Model file for the job. Use its own axes, mm. Face numbers are marked on the shaded views. A direction names the side the tool comes from. Round coordinates to 2 decimals unless told otherwise and drop trailing zeros. Order: outer loops, then holes, each group sorted by start corner. A loop starts at its lowest first (then second) coordinate and runs counter-clockwise, first axis right, second up. Notation, with made-up numbers: (56, 72) - (89, 72) arc R29 cw to (89, 96) - close; hole circle Ø7 at (-27.5, -22.5). An arc over 180 degrees is marked (long way). Answer as CSV lines item,"result". Start each with the question number.
1. Band-saw the part on B-B on y = 3.75. List the corners of the cut face in (x, z), then the cut area to 3 significant figures.
2. Pin check, flat tips, straight feed: pin 1 Ø6 at (x, y) = (2, -1.5) entering from +Z; pin 2 Ø1.5 at (x, y) = (-2.5, 1) entering from +Z. Stop position of each tip, or through.
3. Band-saw the part on C-C on z = 10.25. List the corners of the cut face in (x, y), then the cut area to 3 significant figures.
4. Band-saw the part on A-A on z = 8. List the corners of the cut face in (x, y).
5. Band-saw the part on D-D on x = -3.5. List the corners of the cut face in (y, z), then the cut area to 3 significant figures.
6. Wall check: line 1 along Y through (x, z) = (0, 9.8); line 2 along Y through (x, z) = (1, 7.5); line 3 along X through (y, z) = (0, 9.7). Give the ranges that are in metal, low to high. Write a range as [from, to].
7. Pull direction Y, two halves, no side cores. Call the marked faces 1, 2 and 3: released by +Y, released by -Y, zero draft, split by the parting line, or undercut.
8. 3-axis set-ups, long thin cutter, end or side, ignore diameter. For the marked faces 4 and 5: which of +Z, -Z, +X, -X, +Y, -Y reach the whole face in a straight line?
```python
from build123d import *

# Parameters (mm, degrees)
F0_W          = 10
F0_H          = 10
F1_DEPTH      = 25
F1_DEPTH_BACK = 5
F4_W          = 10
F4_H          = 5.4510665399
F5_DEPTH      = 25
F5_DEPTH_BACK = 25


with BuildPart() as f1:
    # F0 (on Top) → F1 (new body, two sides)
    with BuildSketch(Plane.XY) as f1_sk:
        Rectangle(F0_W, F0_H)
    extrude(amount=F1_DEPTH)
    extrude(f1_sk.sketch, amount=-F1_DEPTH_BACK)

    # F2 (on Front) → F3 (revolve, cut)
    with BuildSketch(Plane.XZ):
        Polygon((2.55, 8.6417774172), (2.55, 25), (0, 25), (0, 5), align=None)
    revolve(axis=Axis((0, 0, 15), (0, 0, -1)), mode=Mode.SUBTRACT)

    # F4 (on Front) → F5 (cut, two sides)
    with BuildSketch(Plane.XZ) as f5_sk:
        with BuildLine():
            ThreePointArc((-5, 11.7330665399), (0.3429792874, 10.3044447979), (5, 7.3210665399))
            Line((5, 7.3210665399), (5, 25))
            Line((5, 25), (-5, 25))
            Line((-5, 25), (-5, 11.7330665399))
        make_face()
        with Locations((0, -2.2744667301)):
            Rectangle(F4_W, F4_H)
    extrude(amount=-F5_DEPTH, mode=Mode.SUBTRACT)
    extrude(f5_sk.sketch, amount=F5_DEPTH_BACK, mode=Mode.SUBTRACT)


solid = f1.part
```
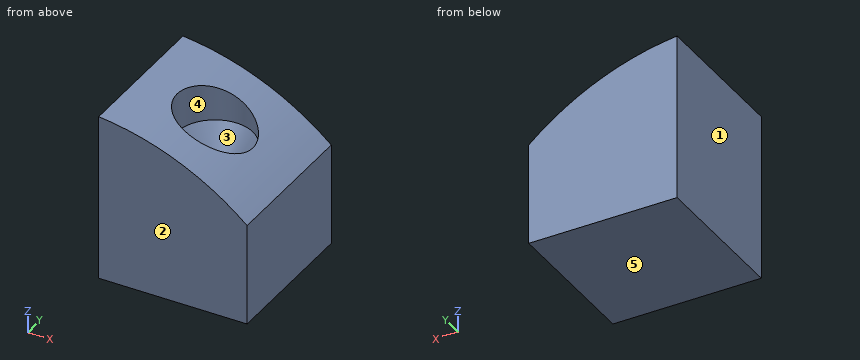
Reply:
1,outline,"(-5, 0.45) - (5, 0.45) - (5, 7.32) arc R18 ccw to (-5, 11.73) - close"
1,area,"97.0 mm2"
2,pin 1,"stops at z = 10.78"
2,pin 2,"stops at z = 11.46"
3,outline,"(-5, -5) - (0.47, -5) - (0.47, -2.51) arc R2.55 cw (long way) to (0.47, 2.51) - (0.47, 5) - (-5, 5) - close"
3,area,"42.1 mm2"
4,outline,"(-5, -5) - (4.18, -5) - (4.18, 5) - (-5, 5) - close; hole circle Ø4.2 at (0, 0)"
5,outline,"(-5, 0.45) - (5, 0.45) - (5, 11.51) - (-5, 11.51) - close"
5,area,"111 mm2"
6,line 1,"y = [-5, -2.55], [2.55, 5]"
6,line 2,"y = [-5, -1.44], [1.44, 5]"
6,line 3,"x = [-5, -2.55]"
7,face 1,"zero draft"
7,face 2,"released by -Y"
7,face 3,"undercut"
8,face 4,"+Z"
8,face 5,"-Z, +X, -X, +Y, -Y"
